Input: dimensioned drawing with shaded views. Units: mm. Origin: part minimum x, y, z. Round coordinates to 2 decimals unless told otherwise and drop trailing zeros. Loops run counter-clockwise (first coordinate to the right, second up) from the corner with the lowest first, then second, coordinate; pieces in that order, holes last. Notation, with made-up numbers: (29, 3) - (48, 3) arc R27 ccw to (48, 29) - close; hole circle Ø10 at (33, 80.5). An arc over 180 degrees is marked (long way). One line per question, with ' | ' between items.
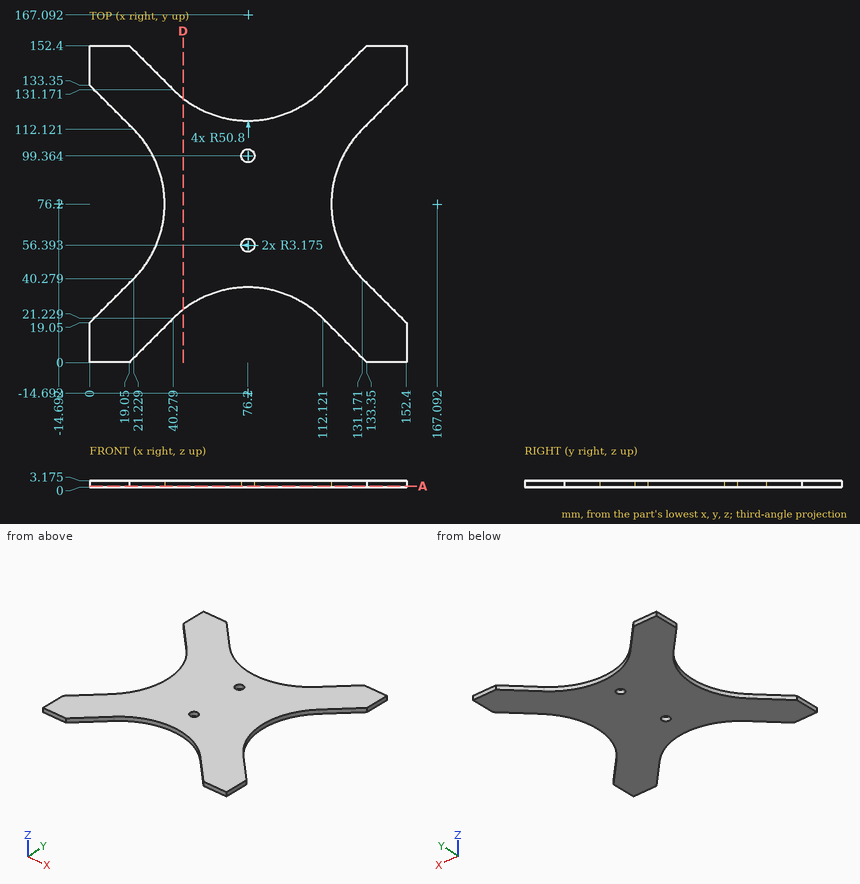
1. Material intervals for probe 1 along Y at (x, z) = (140.5, 2.65); probe 2 along X at (y, z) = (17, 2.4); probe 3 along X at (y, z) = (26, 1.8), sorted ascending.
Worked out:
probe 1: y = 0 to 30.95, 121.45 to 152.4 | probe 2: x = 0 to 36.05, 116.35 to 152.4 | probe 3: x = 6.95 to 45.79, 106.61 to 145.45
2. Section query A-A, the plane z = 0.5. Give the number of separate pieces and of enclosed holes in the cut face, plus the area to 3 significant figures.
Worked out:
separate pieces: 1 | enclosed holes: 2 | area: 12,300 mm2
3. Contact query for flat-ended pins moving along their axis: P1, Ø1.5, axis at y = 57.5, z = 2, coming from the +X side; P2, Ø1.5, axis at y = 70.5, z = 2, coming from the -X side. Output: stop coordinate, or through.
Worked out:
P1: stops at x = 120.16 | P2: stops at x = 35.7
4. Section query D-D, the plane x = 45. Return loops of the section in (y, z) (1 decimal).
Worked out:
outline: (25.4, 0) - (127, 0) - (127, 3.2) - (25.4, 3.2) - close
